Build history of the part. All positions in model axes, mm. A direction names the side the tool comes from. Round coordinates to 2 decimals unless told otherwise and drop trailing zeros. Write each loop counter-clockwise with the first axis right and the second up, starting at its lowest first coordinate (ties: lowest second). Pieces come first, ordered by that corner, then holes. Notation, with made-up numbers: (53.5, 66) - (91.5, 66) arc R37 cw to (91.5, 104) - close; hole circle Ø9 at (-9, -23.75). An arc over 180 degrees is marked (long way). Answer as a JSON object with one key per item and string values. Group by question number.
Item 1: Probe line 1 (X direction, y = 5.5, z = 21.25); line 2 (X direction, y = 3.5, z = 22.5); line 3 (Z direction, x = -47.5, y = 5.25). List the from-to ranges inside material, lowest first. Write a range as from..to.
Item 2: Which spindle directions (+Z, -Z, +X, -X, +Y, -Y) get a long thin tool onto all of the face, cutting with end or side? Do faces 5 (the cylindrical face through (-22.898, 3.219, 4.816)), 6 (the cylindrical face through (-26.141, 3.219, 29.077)), 7 (the cylindrical face through (-32.623, 3.131, 13.721)). Say none if no direction does.
Item 3: Two-plate mould, pull along X, no slides. Class faces 1 (the flat face through (2.176, 3, 17)), 2 (the cylindrical face through (-43.428, 3.131, 22.925)), 3 (the flat face through (-51.164, 3, 17)), 4 (the flat face through (-25, 0, 17)): +X half, -X half, draft (parallel to the pull), parting line (faces both ways), or undercut.
Item 4: Slice it at B-B, the plane y = 4. List the corners of the cut face in (x, z) (3 decimals), then the cut area to 3 significant figures.
Item 5: Flat gauge pins, fed straight in: pin 1 (6 mm diameter, centred on x = -14.76, z = 21.17, fed in from +Y); pin 2 (3 mm diameter, centred on x = -23, y = 1.5, fed in from +Z). Where does each tip first touch, or does it go through?
Item 6: Slice it at A-A, the plane z = 20.75. List the corners of the cut face in (x, y), then the cut area to 3 significant figures.
from build123d import *

# Parameters (mm, degrees)
SKETCH1_R           = 1.905
BOSS_EXTRUDE1_DEPTH = 6.35
FILLET1_R           = 3.81


with BuildPart() as part:
    # Sketch1 → Boss-Extrude1 (new body)
    with BuildSketch(Plane(origin=(0, 0, 0), x_dir=(1, 0, 0), z_dir=(0, 1, 0))):
        Polygon((-51.164237676, -4.231087287), (-51.164237676, -29.631087287), (-25.764237676, -29.631087287), (-24.494237676, -27.091087287), (-23.224237676, -29.631087287), (2.175762324, -29.631087287), (2.175762324, -4.231087287), (-23.224237676, -4.231087287), (-24.494237676, -6.771087287), (-25.764237676, -4.231087287), align=None)
        with Locations(Location((-42.698849573, -21.165699184, 0), (0, 0, 270))):
            Circle(SKETCH1_R, mode=Mode.SUBTRACT)
        with Locations(Location((-34.22962578, -12.696475391, 0), (0, 0, 270))):
            Circle(SKETCH1_R, mode=Mode.SUBTRACT)
        with Locations(Location((-14.758849573, -21.165699184, 0), (0, 0, 270))):
            Circle(SKETCH1_R, mode=Mode.SUBTRACT)
        with Locations(Location((-6.28962578, -12.696475391, 0), (0, 0, 270))):
            Circle(SKETCH1_R, mode=Mode.SUBTRACT)
    extrude(amount=BOSS_EXTRUDE1_DEPTH)

    # Fillet1
    fillet1_edges = [part.edges().sort_by_distance(p)[0] for p in [
        (-51.164237676, 3.175, 29.631087287),
        (-51.164237676, 3.175, 4.231087287),
        (-25.764237676, 3.175, 4.231087287),
        (-23.224237676, 3.175, 4.231087287),
        (2.175762324, 3.175, 4.231087287),
        (2.175762324, 3.175, 29.631087287),
        (-23.224237676, 3.175, 29.631087287),
        (-25.764237676, 3.175, 29.631087287),
    ]]
    fillet(fillet1_edges, radius=FILLET1_R)


solid = part.part
Geometry says:
{
 "1": {"line 1": "x = -51.16..-44.6, -40.8..-16.66, -12.86..2.18", "line 2": "x = -51.16..-44.06, -41.34..-16.12, -13.4..2.18", "line 3": "z = 4.23..29.63"},
 "2": {"face 5": "-Z, +Y, -Y", "face 6": "+Z, +Y, -Y", "face 7": "+Y, -Y"},
 "3": {"face 1": "+X half", "face 2": "undercut", "face 3": "-X half", "face 4": "draft"},
 "4": {"outline": "(-51.164, 8.041) arc R3.81 ccw to (-47.354, 4.231) - (-28.119, 4.231) arc R3.81 ccw to (-24.711, 6.337) - (-24.494, 6.771) - (-24.277, 6.337) arc R3.81 ccw to (-20.87, 4.231) - (-1.634, 4.231) arc R3.81 ccw to (2.176, 8.041) - (2.176, 25.821) arc R3.81 ccw to (-1.634, 29.631) - (-20.87, 29.631) arc R3.81 ccw to (-24.277, 27.525) - (-24.494, 27.091) - (-24.711, 27.525) arc R3.81 ccw to (-28.119, 29.631) - (-47.354, 29.631) arc R3.81 ccw to (-51.164, 25.821) - close; hole circle Ø3.81 at (-42.699, 21.166); hole circle Ø3.81 at (-34.23, 12.696); hole circle Ø3.81 at (-14.759, 21.166); hole circle Ø3.81 at (-6.29, 12.696)", "area": "1,290 mm^2"},
 "5": {"pin 1": "stops at y = 6.35", "pin 2": "stops at z = 29.58"},
 "6": {"outline": "(-51.16, 0) - (-44.56, 0) - (-44.56, 6.35) - (-51.16, 6.35) - close; (-40.84, 0) - (-16.62, 0) - (-16.62, 6.35) - (-40.84, 6.35) - close; (-12.9, 0) - (2.18, 0) - (2.18, 6.35) - (-12.9, 6.35) - close", "area": "291 mm^2"}
}
